Verification items for the finished model (mm, model axes). A direction names the side the tool comes from. Coordinates: 2 decimals unless noted, no trailing zeros. Order: outer loops, then holes, each group sorted by start corner. A loop starts at its lowest first (then second) coordinate and runs counter-clockwise, first axis right, second up. Notation, with made-up numbers: (33.5, 89) - (76.5, 89) arc R31 ccw to (76.5, 125) - close; hole circle Ø4 at (-30, 8.5). An arc over 180 degrees is marked (long way). Answer as CSV lines item,"result". Start each with the question number.
1. Material ranges on L1, parallel to Y at x = -2, z = 16; L2, parallel to Z at x = 0, y = -59; L3, parallel to Y at x = 14, z = 80, recorded low to high. Write a range as [from, to].
2. Section check D-D (z = 52). Record the cut outline in (x, y), and give its area (3 significant figures).
3. Section check B-B (x = 0). Record the cut outline in (y, z), and give its area (3 significant figures).
4. Section check C-C (y = 51.5). Record the cut outline in (x, z).
5. Go/stop test with flat-tipped pins: pin 1 (20 mm diameter, centred on x = -1, z = 42.5, fed in from -Y); pin 2 (1 mm diameter, centred on x = -29.5, z = 67, fed in from -Y). Record where each tip stops, or that it passes through.
6. Mould release check, pull along X, two halves, no side actions. Record for faces 1 (the flat face through (0, -53, 15)), 2 (the cylindrical face through (29.05, -63.27, 80.93)), 3 (the flat face through (40, 14, 49)), 4 (the flat face through (-1, 95, 49)): pulls with the +X half, pulls with the -X half, needs draft (parallel to the pull), parting line crosses it, or undercut.
7. Set-up check for faces 5 (the flat face through (33, -63, 52)), 6 (the flat face through (-29.563, 17.006, 46.342)), 7 (the flat face through (-30, 21, 0)): record each of +Z, -Z, +X, -X, +Y, -Y from which the full face is reachable in a straight line by a thin tool's end or side.
8. Section check A-A (z = 16.5). Record the cut outline in (x, y).
from build123d import *

# Parameters (mm, degrees)
F0_W     = 80
F0_H     = 160
F1_DEPTH = 100
F3_DEPTH = 94
F5_DEPTH = 3.5
F6_R     = 31
F7_DEPTH = 25
F8_ANGLE = 180


with BuildPart() as f1:
    # F0 (on Top) → F1 (new body)
    with BuildSketch(Plane.XY):
        with Locations((0, 15)):
            Rectangle(F0_W, F0_H)
    extrude(amount=F1_DEPTH)

    # F2 (on face) → F3 (cut)
    with BuildSketch(Plane(origin=(0, 0, 0), x_dir=(1, 0, 0), z_dir=(0, 0, -1))):
        Polygon((-25, -89), (25, -89), (34, 53), (-34, 53), align=None)
    extrude(amount=-F3_DEPTH, mode=Mode.SUBTRACT)

    # F4 (on face) → F5 (cut)
    with BuildSketch(Plane.XZ.offset(65)):
        with BuildLine():
            Line((24.33105, 85), (-24.33105, 85))
            ThreePointArc((-24.33105, 85), (-28.991378, 80.991378), (-33, 76.33105))
            Line((-33, 76.33105), (-33, 27.66895))
            ThreePointArc((-33, 27.66895), (-28.991378, 23.008622), (-24.33105, 19))
            Line((-24.33105, 19), (24.33105, 19))
            ThreePointArc((24.33105, 19), (28.991378, 23.008622), (33, 27.66895))
            Line((33, 27.66895), (33, 76.33105))
            ThreePointArc((33, 76.33105), (28.991378, 80.991378), (24.33105, 85))
        make_face()
    extrude(amount=-F5_DEPTH, mode=Mode.SUBTRACT)

    # F6 (on face) → F7 (cut)
    with BuildSketch(Plane.XZ.offset(61.5)):
        with Locations((0, 52)):
            Circle(F6_R)
    extrude(amount=-F7_DEPTH, mode=Mode.SUBTRACT)


with BuildPart() as f8_1:
    # F8: copy of F1
    add(f1.part.rotate(Axis((40, 15, 0), (0, -1, 0)), F8_ANGLE))


solid = f1.part
Evaluation:
1,L1,"y = [-65, -53], [89, 95]"
1,L2,"z = [0, 21], [83, 100]"
1,L3,"y = [-61.5, -53], [89, 95]"
2,outline,"(-40, -65) - (-33, -65) - (-33, -61.5) - (-31, -61.5) - (-31, -53) - (-34, -53) - (-25, 89) - (25, 89) - (34, -53) - (31, -53) - (31, -61.5) - (33, -61.5) - (33, -65) - (40, -65) - (40, 95) - (-40, 95) - close"
2,area,"3,660 mm²"
3,outline,"(-65, 0) - (-53, 0) - (-53, 21) - (-61.5, 21) - (-61.5, 19) - (-65, 19) - close; (-65, 85) - (-61.5, 85) - (-61.5, 83) - (-53, 83) - (-53, 94) - (89, 94) - (89, 0) - (95, 0) - (95, 100) - (-65, 100) - close"
3,area,"1,890 mm²"
4,outline,"(-40, 0) - (-27.38, 0) - (-27.38, 94) - (27.38, 94) - (27.38, 0) - (40, 0) - (40, 100) - (-40, 100) - close"
5,pin 1,"stops at y = 89"
5,pin 2,"stops at y = -61.5"
6,face 1,"undercut"
6,face 2,"undercut"
6,face 3,"pulls with the +X half"
6,face 4,"needs draft"
7,face 5,"-Y"
7,face 6,"-Z"
7,face 7,"-Z, +X, -X, +Y, -Y"
8,outline,"(-40, -65) - (40, -65) - (40, 95) - (-40, 95) - close; hole (-34, -53) - (34, -53) - (25, 89) - (-25, 89) - close"
